```python
from build123d import *

# Parameters (mm, degrees)
SKETCH1_W           = 30
SKETCH1_H           = 15
BOSS_EXTRUDE1_DEPTH = 20
SKETCH2_W           = 8.2
SKETCH2_H           = 5
CUT_EXTRUDE1_DEPTH  = 21
SKETCH3_R           = 2.75
CUT_EXTRUDE2_DEPTH  = 16
BOSS_EXTRUDE2_REACH = 9.5
SKETCH5_W           = 30
SKETCH5_H           = 15
BOSS_EXTRUDE3_DEPTH = 20
SKETCH6_W           = 30
SKETCH6_H           = 5
BOSS_EXTRUDE4_DEPTH = 2
SKETCH7_R           = 2.75
CUT_EXTRUDE3_DEPTH  = 18
SKETCH8_R           = 5
CUT_EXTRUDE4_DEPTH  = 10
SKETCH10_R          = 6
CUT_EXTRUDE5_DEPTH  = 2
BOSS_EXTRUDE5_DEPTH = 15
SKETCH12_W          = 10
SKETCH12_H          = 20
CUT_EXTRUDE6_DEPTH  = 15


with BuildPart() as part:
    # Sketch1 → Boss-Extrude1 (new body)
    with BuildSketch(Plane.XY):
        with Locations((15, 7.5)):
            Rectangle(SKETCH1_W, SKETCH1_H)
    extrude(amount=BOSS_EXTRUDE1_DEPTH)

    # Sketch2 → Cut-Extrude1 (cut, through all)
    with BuildSketch(Plane.XY.offset(20)):
        with Locations((15, 10)):
            Rectangle(SKETCH2_W, SKETCH2_H)
    extrude(amount=-CUT_EXTRUDE1_DEPTH, mode=Mode.SUBTRACT)

    # Sketch3 → Cut-Extrude2 (cut, through all)
    with BuildSketch(Plane(origin=(0, 15, 0), x_dir=(1, 0, 0), z_dir=(0, 1, 0))):
        with Locations((15, -10)):
            Circle(SKETCH3_R)
    extrude(amount=-CUT_EXTRUDE2_DEPTH, mode=Mode.SUBTRACT)

    # Sketch4 → Boss-Extrude2 (add, up to next)
    with BuildSketch(Plane(origin=(0, 7.5, 0), x_dir=(1, 0, 0), z_dir=(0, 1, 0)), mode=Mode.PRIVATE) as boss_extrude2_sk1:
        Polygon((19.1, -7.5), (15.1, -5.133920143), (10.9, -7.5), (10.9, 0), (19.1, 0), align=None)
    boss_extrude2_tool1 = extrude(boss_extrude2_sk1.sketch, amount=BOSS_EXTRUDE2_REACH, mode=Mode.PRIVATE) - part.part
    add(boss_extrude2_tool1.solids().sort_by_distance((14.993757, 7.5, 3.195407))[0])

    # Sketch5 → Boss-Extrude3 (add)
    with BuildSketch(Plane(origin=(0, 0, 0), x_dir=(-1, 0, 0), z_dir=(0, 0, -1))):
        with Locations((0, 7.5)):
            Rectangle(SKETCH5_W, SKETCH5_H)
    extrude(amount=BOSS_EXTRUDE3_DEPTH)

    # Sketch6 → Boss-Extrude4 (add)
    with BuildSketch(Plane.XZ):
        with Locations((0, -10)):
            Rectangle(SKETCH6_W, SKETCH6_H)
    extrude(amount=BOSS_EXTRUDE4_DEPTH)

    # Sketch7 → Cut-Extrude3 (cut, through all)
    with BuildSketch(Plane(origin=(0, 15, 0), x_dir=(1, 0, 0), z_dir=(0, 1, 0))):
        with Locations((7.5, 10)):
            Circle(SKETCH7_R)
        with Locations((-7.5, 10)):
            Circle(SKETCH7_R)
    extrude(amount=-CUT_EXTRUDE3_DEPTH, mode=Mode.SUBTRACT)

    # Sketch8 → Cut-Extrude4 (cut)
    with BuildSketch(Plane(origin=(0, 15, 0), x_dir=(1, 0, 0), z_dir=(0, 1, 0))):
        with Locations((7.5, 10)):
            Circle(SKETCH8_R)
        with Locations((-7.5, 10)):
            Circle(SKETCH8_R)
    extrude(amount=-CUT_EXTRUDE4_DEPTH, mode=Mode.SUBTRACT)

    # Sketch10 → Cut-Extrude5 (cut)
    with BuildSketch(Plane.XZ.offset(2)):
        with Locations((-7.5, -10)):
            Circle(SKETCH10_R)
        with Locations((7.5, -10)):
            Circle(SKETCH10_R)
    extrude(amount=-CUT_EXTRUDE5_DEPTH, mode=Mode.SUBTRACT)

    # Sketch11 → Boss-Extrude5 (add)
    with BuildSketch(Plane(origin=(0, 15, 0), x_dir=(1, 0, 0), z_dir=(0, 1, 0))):
        Polygon((-15, 0), (0, -20), (0, 0), align=None)
    extrude(amount=-BOSS_EXTRUDE5_DEPTH)

    # Sketch12 → Cut-Extrude6 (cut)
    with BuildSketch(Plane(origin=(0, 15, 0), x_dir=(1, 0, 0), z_dir=(0, 1, 0))):
        with Locations((25, -10)):
            Rectangle(SKETCH12_W, SKETCH12_H)
    extrude(amount=-CUT_EXTRUDE6_DEPTH, mode=Mode.SUBTRACT)


solid = part.part
```
Geometry check sheet. Reference: the model listing, model coordinates, mm. A direction names the side the tool comes from. Round coordinates to 2 decimals unless told otherwise and drop trailing zeros. Loops run counter-clockwise (first coordinate to the right, second up) from the corner with the lowest first, then second, coordinate; pieces in that order, holes last. Notation, with made-up numbers: (-4, -16.5) - (0, -16.5) arc R28 ccw to (0, 19.5) - close; hole circle Ø6 at (-35.5, 65). An arc over 180 degrees is marked (long way). Use a Markdown table: item, result.
Q1. Go/stop test with flat-tipped pins: P1, Ø1, axis at y = 4.5, z = 5.5, coming from the -X side; P2, Ø8, axis at x = -7.5, z = -10, coming from the -Y side; P3, Ø2.5, axis at y = 10, z = 13, coming from the -X side. Record where each tip stops, or that it passes through.
Solutions:
| item | result |
|---|---|
| P1 | stops at x = -11.25 |
| P2 | stops at y = 0 |
| P3 | stops at x = -6.19 |
Q2. Material ranges on line 1 (X direction, y = 9, z = -10); line 2 (X direction, y = 2.1, z = -10); line 3 (Y direction, x = 11, z = -1), recorded low to high.
Solutions:
| item | result |
|---|---|
| line 1 | x = -15 to -12.5, -2.5 to 2.5, 12.5 to 15 |
| line 2 | x = -15 to -10.25, -4.75 to 4.75, 10.25 to 15 |
| line 3 | y = 0 to 15 |
Q3. Cross-section at B-B on z = 15. Record the cut outline in (x, y), plus the area to 3 significant figures.
Solutions:
| item | result |
|---|---|
| outline | (-3.75, 0) - (20, 0) - (20, 15) - (-3.75, 15) - close; hole (10.9, 7.5) - (19.1, 7.5) - (19.1, 12.5) - (10.9, 12.5) - close |
| area | 315 mm2 |
Q4. Access from +Z, -Z, +X, -X, +Y, -Y to the whole of each face (thin tool, end or side, straight path). Record for faces 4 (the flat face through (-5, 5, -8)), 5 (the flat face through (-14, -1, -12.5)), 6 (the flat face through (0, -1, -7.5)), 7 (the flat face through (19.1, 10, 14)).
Solutions:
| item | result |
|---|---|
| face 4 | +Y |
| face 5 | -Z, +X, -X, -Y |
| face 6 | +Z, +X, -X, -Y |
| face 7 | +Z |
Q5. Cross-section at C-C on x = 7.5. Record the cut outline in (y, z).
Solutions:
| item | result |
|---|---|
| outline | (0, -20) - (15, -20) - (15, -15) - (5, -15) - (5, -12.75) - (0, -12.75) - close; (0, -7.25) - (5, -7.25) - (5, -5) - (15, -5) - (15, 20) - (0, 20) - close |
Q6. Draft check along Z on faces 1 (the flat face through (0, -1, -12.5)), 2 (the cylindrical face through (12.253, 3.802, 9.879)), 3 (the flat face through (17.128, 9.965, 6.334)). Enter one of: released by +Z, released by -Z, zero draft, split by the parting line, or undercut.
Solutions:
| item | result |
|---|---|
| face 1 | released by -Z |
| face 2 | undercut |
| face 3 | released by +Z |
Q7. Cross-section at A-A on y = 1.25. Record the cut outline in (x, z), plus the area to 3 significant figures.
Solutions:
| item | result |
|---|---|
| outline | (-15, -20) - (15, -20) - (15, 0) - (20, 0) - (20, 20) - (0, 20) - (-15, 0) - close; hole circle Ø5.5 at (-7.5, -10); hole circle Ø5.5 at (7.5, -10); hole circle Ø5.5 at (15, 10) |
| area | 1,080 mm2 |
Q8. Cross-section at D-D on y = 12. Record the cut outline in (x, z).
Solutions:
| item | result |
|---|---|
| outline | (-15, -20) - (15, -20) - (15, 0) - (20, 0) - (20, 20) - (19.1, 20) - (19.1, 7.5) - (15.1, 5.13) - (10.9, 7.5) - (10.9, 20) - (0, 20) - (-15, 0) - close; hole circle Ø10 at (-7.5, -10); hole circle Ø10 at (7.5, -10) |
